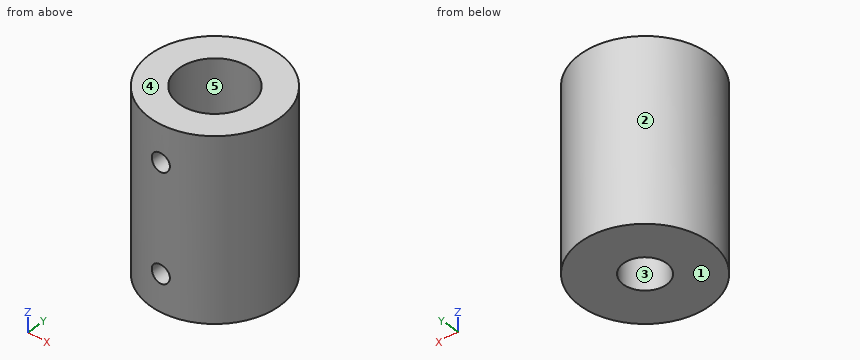
from build123d import *

# Parameters (mm, degrees)
SKETCH1_R           = 9
SKETCH1_R_2         = 3
BOSS_EXTRUDE1_DEPTH = 25
SKETCH2_R           = 5
CUT_EXTRUDE1_DEPTH  = 12.446
SKETCH3_R           = 1.27
CUT_EXTRUDE2_DEPTH  = 12.446


with BuildPart() as part:
    # Sketch1 → Boss-Extrude1 (new body)
    with BuildSketch(Plane.XY):
        Circle(SKETCH1_R)
        Circle(SKETCH1_R_2, mode=Mode.SUBTRACT)
    extrude(amount=BOSS_EXTRUDE1_DEPTH)

    # Sketch2 → Cut-Extrude1 (cut)
    with BuildSketch(Plane.XY.offset(25)):
        Circle(SKETCH2_R)
    extrude(amount=-CUT_EXTRUDE1_DEPTH, mode=Mode.SUBTRACT)

    # Sketch3 → Cut-Extrude2 (cut)
    with BuildSketch(Plane(origin=(0, 0, 0), x_dir=(1, 0, 0), z_dir=(0, 1, 0))):
        with Locations((0, -5.08)):
            Circle(SKETCH3_R)
        with Locations((0, -19.92)):
            Circle(SKETCH3_R)
    extrude(amount=-CUT_EXTRUDE2_DEPTH, mode=Mode.SUBTRACT)


solid = part.part
Work out the finished part from the listing and answer in its coordinate system (mm). Face numbers are marked on the shaded views. A direction names the side the tool comes from. Coordinates: 2 decimals unless noted, no trailing zeros. Write each loop counter-clockwise with the first axis right and the second up, starting at its lowest first coordinate (ties: lowest second). Pieces come first, ordered by that corner, then holes. Notation, with made-up numbers: M 39.5,-7 L 85.5,-7 A7 ccw 85.5,5 Z; hole C -8.5,-30 d2. An arc over 180 degrees is marked long. Answer as CSV lines item,"result". Start each with the question number.
Item 1: Section C-C on z = 2.25 is taken. Write down the section's boundary in (x, y).
Item 2: Flat-ended cylindrical pins translate along their axes: P1, Ø4, axis at y = 2, z = 11, coming from the +X side; P2, Ø5, axis at x = -4.5, z = 14, coming from the +Y side; P3, Ø2, axis at x = -5, z = 14, coming from the -Y side; P4, Ø5, axis at x = 0, y = 0, coming from the -Z side. Find the tip coordinate at first contact, or state that the pin passes through.
Item 3: Determine the mould class of the marked faces 1, 2 and 3 for opening direction Y: released by +Y, released by -Y, zero draft, split by the parting line, or undercut.
Item 4: Consider L1, parallel to Z at x = 0, y = -7; L2, parallel to Y at x = 0, z = 7.25; L3, parallel to Z at x = -2, y = 3.75. Determine where each line is inside the solid, lowest interval first.
Item 5: Section B-B on x = 0 is taken. Write down the section's boundary in (y, z).
Item 6: A tool of negligible diameter and unlimited length cuts with its end or side. For the marked faces 4 and 5, from which of +Z, -Z, +X, -X, +Y, -Y can it reach the whole face along a straight path? Write none if from no direction.
Item 7: Section D-D on y = -4.5 is taken. Write down the section's boundary in (x, z), and give its area (3 significant figures).
Item 8: Section A-A on y = 0 is taken. Write down the section's boundary in (x, z).
Checks:
1,outline,"C 0,0 d18; hole C 0,0 d6"
2,P1,"stops at x = 9"
2,P2,"stops at y = 8.77"
2,P3,"stops at y = -8.06"
2,P4,"passes through"
3,face 1,"zero draft"
3,face 2,"split by the parting line"
3,face 3,"undercut"
4,L1,"z = 0 to 3.81, 6.35 to 18.65, 21.19 to 25"
4,L2,"y = -9 to -3, 3 to 9"
4,L3,"z = 0 to 12.55"
5,outline,"M -9,0 L -3,0 L -3,3.81 L -9,3.81 Z; M -9,6.35 L -3,6.35 L -3,12.55 L -5,12.55 L -5,18.65 L -9,18.65 Z; M -9,21.19 L -5,21.19 L -5,25 L -9,25 Z; M 3,0 L 9,0 L 9,25 L 5,25 L 5,12.55 L 3,12.55 Z"
6,face 4,"+Z, +X, -X, +Y, -Y"
6,face 5,"+Z"
7,outline,"M -7.79,0 L 7.79,0 L 7.79,25 L 2.18,25 L 2.18,12.55 L -2.18,12.55 L -2.18,25 L -7.79,25 Z; hole C 0,5.08 d2.54"
7,area,"330 mm²"
8,outline,"M -9,0 L -3,0 L -3,12.55 L -5,12.55 L -5,25 L -9,25 Z; M 3,0 L 9,0 L 9,25 L 5,25 L 5,12.55 L 3,12.55 Z"
